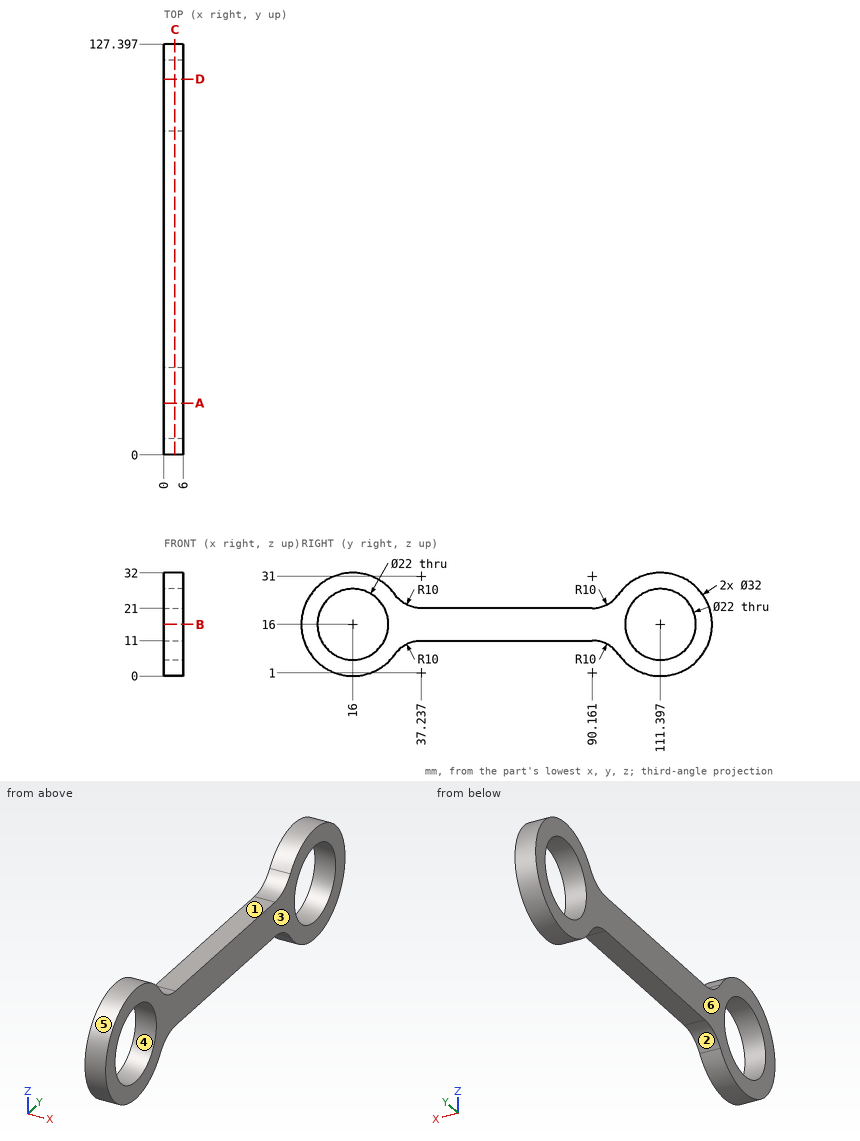
Design review of the part shown in the three views and the two pictorial views. Dimensions are in mm from the part's minimum x, y and z. A direction names the side the tool comes from. Give positions to 0.01 mm unless a question says otherwise; leave off trailing zeros. Write each loop counter-clockwise with the first axis right and the second up, starting at its lowest first coordinate (ties: lowest second). Pieces come first, ordered by that corner, then holes. Notation, with made-up numbers: (4.25, 2) - (29.25, 2) arc R25 cw to (29.25, 40) - close; hole circle Ø5 at (-7.75, 50.25). An arc over 180 degrees is marked (long way). Return JSON: item names as keys, results as strings. Group by question number.
(1) To check wall thickness, follow probe 1 along Y at (x, z) = (2.15, 16); probe 2 along Y at (x, z) = (4, 25) (1 decimal); probe 3 along Y at (x, z) = (2.35, 9.5) (1 decimal). State the ranges of each line that lie inside material, in increasing order.
(2) We need section D-D, the plane y = 116.5. Give the boundary of the cut face in (x, z) (1 decimal).
(3) Insertion check: pin 1 (1.8 mm diameter, centred on x = 3.5, y = 53, fed in from +Z); pin 2 (3 mm diameter, centred on y = 42.5, z = 23.5, fed in from -X); pin 3 (2 mm diameter, centred on x = 1, y = 109, fed in from -Z); pin 4 (3 mm diameter, centred on x = 4, z = 26, fed in from -Y) (1 decimal). Each pin has a flat end and moves straight along its axis. Give the tip position at first contact, or say it passes through.
(4) Machinability: for the marked faces 1, 2 and 3, which of the approach directions +Z, -Z, +X, -X, +Y, -Y give a long, thin tool a straight path to every point of the face, cutting with its end or side? Answer none if there is none.
(5) We need section A-A, the plane y = 16. Give the boundary of the cut face in (x, z), then the cut area to 3 significant figures.
(6) We need section B-B, the plane z = 16. Give the boundary of the cut face in (x, y).
(7) We need section C-C, the plane x = 3.4. Give the boundary of the cut face in (y, z), then the cut area to 3 significant figures.
(8) Mouldability with a two-part tool opening along Y and no side actions: class the marked faces 4, 5 and 6 as +Y half, -Y half, draft (parallel to the pull), parting line (faces both ways), or undercut.
Reported:
{
 "1": {"probe 1": "y = 0 to 5, 27 to 100.4, 122.4 to 127.4", "probe 2": "y = 2.8 to 9.7, 22.3 to 29.2, 98.2 to 105.1, 117.7 to 124.6", "probe 3": "y = 1.4 to 7.1, 24.9 to 32, 95.4 to 102.5, 120.3 to 126"},
 "2": {"outline": "(0, 0.8) - (6, 0.8) - (6, 6.3) - (0, 6.3) - close; (0, 25.7) - (6, 25.7) - (6, 31.2) - (0, 31.2) - close"},
 "3": {"pin 1": "stops at z = 21", "pin 2": "passes through", "pin 3": "stops at z = 0.06", "pin 4": "stops at y = 2.4"},
 "4": {"face 1": "+Z, +X, -X", "face 2": "-Z, +X, -X", "face 3": "+Z, -Z, +X, +Y, -Y"},
 "5": {"outline": "(0, 0) - (6, 0) - (6, 5) - (0, 5) - close; (0, 27) - (6, 27) - (6, 32) - (0, 32) - close", "area": "60.0 mm2"},
 "6": {"outline": "(0, 0) - (6, 0) - (6, 5) - (0, 5) - close; (0, 27) - (6, 27) - (6, 100.4) - (0, 100.4) - close; (0, 122.4) - (6, 122.4) - (6, 127.4) - (0, 127.4) - close"},
 "7": {"outline": "(29.07, 6.77) arc R10 cw to (37.24, 11) - (90.16, 11) arc R10 cw to (98.33, 6.77) arc R16 ccw (long way) to (98.33, 25.23) arc R10 cw to (90.16, 21) - (37.24, 21) arc R10 cw to (29.07, 25.23) arc R16 ccw (long way) to start; hole circle Ø22 at (16, 16); hole circle Ø22 at (111.4, 16)", "area": "1,510 mm2"},
 "8": {"face 4": "undercut", "face 5": "undercut", "face 6": "draft"}
}
